The listing builds one solid part. Answer for the finished solid, in the listing's coordinates (mm). A direction names the side the tool comes from. Give positions to 0.01 mm unless a question says otherwise; leave off trailing zeros. Order: outer loops, then holes, each group sorted by start corner. A loop starts at its lowest first (then second) coordinate and runs counter-clockwise, first axis right, second up. Notation, with made-up numbers: (26, 17) -> (44, 17) arc R25 ccw to (44, 55) -> close; hole circle Ø3 at (-7, 37.5). An arc over 180 degrees is marked (long way). Answer as a JSON object with one key per item and string values. Group by question number.
Autodesk Inventor part; units mm, degrees
ref_plane "YZ Plane" through (0, 0, 0) normal (1, 0, 0) x (0, 1, 0)
ref_plane "XZ Plane" through (0, 0, 0) normal (0, 1, 0) x (-1, 0, 0)
ref_plane "XY Plane" through (0, 0, 0) normal (0, 0, 1) x (1, 0, 0)
sketch "Sketch1" plane through (0, 0, 0) normal (0, 0, 1) x (1, 0, 0)
  line L0 (-150, 125) -> (150, 125)
  line L1 (150, 125) -> (150, -125)
  line L2 (150, -125) -> (-150, -125)
  line L3 (-150, -125) -> (-150, 125)
  point P0 (0, 0)
  point P1 (0, 125)
  point P2 (150, 0)
  dimension "d0" = 300
  dimension "d1" = 250
extrude "Extrusion1" add sketch "Sketch1" along normal blind 39.37
sketch "Sketch2" plane through (0, 0, 39.37) normal (0, 0, 1) x (1, 0, 0)
  line L0 (-150, 125) -> (-150, -125)
  line L1 (150, 125) -> (-150, 125) construction
  line L2 (0, 125) -> (0, -125) construction
  line L3 (-150, -125) -> (150, -125) construction
  point P0 (0, 0)
  point P1 (-120, 0)
  point P2 (120, 0)
  dimension "d4" = 30
hole "Hole1" at (-120, 0, 39.37) at (120, 0, 39.37) direction (0, 0, -1) diameter 10 end through all
hole "Hole2" at (-120, 0, 39.37) at (120, 0, 39.37) direction (0, 0, -1) diameter 20 depth 10 tip angle 118 countersink diameter 25 countersink angle 82
sketch "Sketch3" plane through (0, 0, 0) normal (0, 0, -1) x (-1, 0, 0)
  line L0 (58.5, -28.5) -> (-58.5, -28.5) construction
  line L1 (-58.5, -28.5) -> (-58.5, 28.5) construction
  line L2 (-58.5, 28.5) -> (58.5, 28.5) construction
  line L3 (58.5, 28.5) -> (58.5, -28.5) construction
  circle A0 centre (36, -11.5) radius 2
  line L4 (0, -28.5) -> (0, 28.5) construction
  line L5 (-58.5, 0) -> (58.5, 0) construction
  circle A1 centre (36, 11.5) radius 2
  circle A2 centre (-36, -11.5) radius 2
  circle A3 centre (-36, 11.5) radius 2
  point P0 (0, 0)
  dimension "d19" = 117
  dimension "d20" = 57
  dimension "d24" = 17
  dimension "d25" = 22.5
hole "Hole3" at (-36, -11.5, 0) at (-36, 11.5, 0) at (36, -11.5, 0) at (36, 11.5, 0) direction (0, 0, 1) diameter 4 end through all
sketch "Sketch4" plane through (0, 0, 39.37) normal (0, 0, 1) x (1, 0, 0)
  circle A0 centre (-36, 11.5) radius 2
  circle A1 centre (36, 11.5) radius 2
  circle A2 centre (36, -11.5) radius 2
  point P0 (0, 0)
  point P1 (-36, -11.3289)
hole "Hole5" at (-36, 11.5, 39.37) at (-36, -11.3289, 39.37) at (36, 11.5, 39.37) at (36, -11.5, 39.37) direction (0, 0, -1) diameter 12 depth 8 tip angle 118
properties part number "TablaInferior"
(1) Which of the six approach directions +Z, -Z, +X, -X, +Y, -Y give full straight-line access (tool end or side, diameter ignored) to faces 1 (the cylindrical face through (41.323, 8.731, 35.314)), 2 (the flat face through (2, -125, 19))?
(2) For a pull along Y with two mould halves and no side action, classify faces 3 (the flat face through (-2, 125, 19)), 4 (the flat face through (-150, -2, 19)), 5 (the conical face through (-125.186, 1.152, 26.554)), 6 (the conical face through (37.521, -9.841, 29.117)) as +Y half, -Y half, draft (parallel to the pull), parting line (faces both ways), or undercut.
(3) A flat-ended cylindrical pin translates along its axis: pin 1 Ø4.5 at (x, y) = (36, -11.5) entering from +Z. Find the tip coordinate at first contact, or state that the pin passes through.
(4) A cutting plane is placed at A-A (x = -120). Determine the outline of the cut face in (y, z), and give its area (3 significant figures).
(5) Find the intervals of material crossed by line 1 along Y through (x, z) = (36, 33.75); line 2 along X through (y, z) = (-11.5, 19.75); line 3 along X through (y, z) = (11, 6), in increasing order. Write a range as [from, to].
(6) A cutting plane is placed at B-B (y = 0). Determine the outline of the cut face in (x, z), and give its area (3 significant figures).
Check sheet entries:
{
 "1": {"face 1": "+Z", "face 2": "+Z, -Z, +X, -X, -Y"},
 "2": {"face 3": "+Y half", "face 4": "draft", "face 5": "undercut", "face 6": "undercut"},
 "3": {"pin 1": "stops at z = 29.12"},
 "4": {"outline": "(-125, 0) -> (-5, 0) -> (-5, 26.37) -> (-10, 29.37) -> (-10, 36.49) -> (-12.5, 39.37) -> (-125, 39.37) -> close; (5, 0) -> (125, 0) -> (125, 39.37) -> (12.5, 39.37) -> (10, 36.49) -> (10, 29.37) -> (5, 26.37) -> close", "area": "9,330 mm2"},
 "5": {"line 1": "y = [-125, -17.5], [-5.5, 5.5], [17.5, 125]", "line 2": "x = [-150, -38], [-34, 34], [38, 150]", "line 3": "x = [-150, -37.94], [-34.06, 34.06], [37.94, 150]"},
 "6": {"outline": "(-150, 0) -> (-125, 0) -> (-125, 26.37) -> (-130, 29.37) -> (-130, 36.49) -> (-132.5, 39.37) -> (-150, 39.37) -> close; (-115, 0) -> (115, 0) -> (115, 26.37) -> (110, 29.37) -> (110, 36.49) -> (107.5, 39.37) -> (-107.5, 39.37) -> (-110, 36.49) -> (-110, 29.37) -> (-115, 26.37) -> close; (125, 0) -> (150, 0) -> (150, 39.37) -> (132.5, 39.37) -> (130, 36.49) -> (130, 29.37) -> (125, 26.37) -> close", "area": "10,800 mm2"}
}
